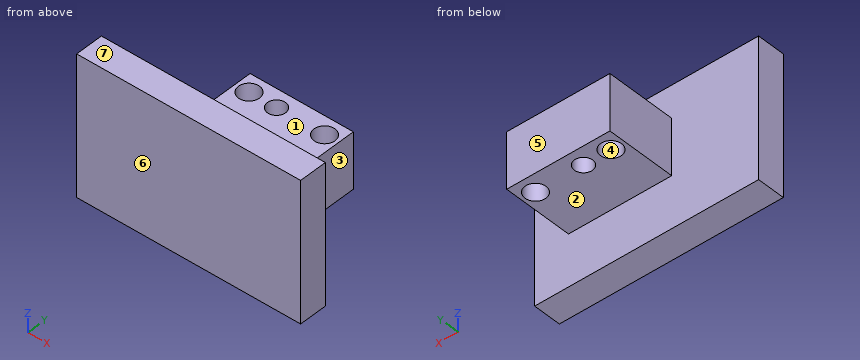
from build123d import *

# Parameters (mm, degrees)
SKETCH1_W           = 80
SKETCH1_H           = 50
MAIN_PLATE_DEPTH    = 10
SKETCH1_3_W         = 36.871622478
SKETCH1_3_H         = 20
BOSS_EXTRUDE2_DEPTH = 25
SKETCH2_R           = 3.760980907
SKETCH2_R_2         = 3.25
CUT_EXTRUDE1_DEPTH  = 20


with BuildPart() as part:
    # Sketch1 → Main Plate (new body)
    with BuildSketch(Plane(origin=(0, 0, 0), x_dir=(1, 0, 0), z_dir=(0, 1, 0))):
        Rectangle(SKETCH1_W, SKETCH1_H)
    extrude(amount=-MAIN_PLATE_DEPTH)

    # Sketch1<3> → Boss-Extrude2 (add)
    with BuildSketch(Plane(origin=(0, 0, 0), x_dir=(1, 0, 0), z_dir=(0, 1, 0))):
        with Locations((9.470325945, -3.44765343)):
            Rectangle(SKETCH1_3_W, SKETCH1_3_H)
    extrude(amount=BOSS_EXTRUDE2_DEPTH)

    # Sketch2 → Cut-Extrude1 (cut)
    with BuildSketch(Plane.XY.offset(13.44765343)):
        with Locations((-4.018286342, 18.961248544)):
            Circle(SKETCH2_R)
        with Locations(Location((22.958938232, 18.961248544, 0), (0, 0, 180))):
            Circle(SKETCH2_R)
        with Locations((5.79860133, 18.961248544)):
            Circle(SKETCH2_R_2)
    extrude(amount=-CUT_EXTRUDE1_DEPTH, mode=Mode.SUBTRACT)


solid = part.part
The listing builds one solid part. Answer for the finished solid, in the listing's coordinates (mm). Face numbers are marked on the shaded views. A direction names the side the tool comes from. Give positions to 0.01 mm unless a question says otherwise; leave off trailing zeros. Order: outer loops, then holes, each group sorted by start corner. A loop starts at its lowest first (then second) coordinate and runs counter-clockwise, first axis right, second up. Notation, with made-up numbers: (85.25, 60) -> (137.25, 60) arc R22 ccw to (137.25, 92) -> close; hole circle Ø11 at (-5.75, 28). An arc over 180 degrees is marked (long way). Put each result on its own line as item: value.
Item 1: For a pull along Y with two mould halves and no side action, classify the marked faces 4, 5, 6 and 7 as released by +Y, released by -Y, zero draft, split by the parting line, or undercut.
Established:
face 4: undercut
face 5: released by +Y
face 6: released by -Y
face 7: zero draft
Item 2: A cutting plane is placed at D-D on x = 14.5. Give the vertices of the cut face in (y, z).
Established:
outline: (-10, -25) -> (0, -25) -> (0, -6.55) -> (25, -6.55) -> (25, 13.45) -> (0, 13.45) -> (0, 25) -> (-10, 25) -> close
Item 3: A cutting plane is placed at A-A on x = -4. Give the vertices of the cut face in (y, z), plus the area to 3 significant figures.
Established:
outline: (-10, -25) -> (0, -25) -> (0, -6.55) -> (15.2, -6.55) -> (15.2, 13.45) -> (0, 13.45) -> (0, 25) -> (-10, 25) -> close; (22.72, -6.55) -> (25, -6.55) -> (25, 13.45) -> (22.72, 13.45) -> close
area: 850 mm^2
Item 4: Straight lines are drawn through the part: line 1 (X direction, y = 7.5, z = 9); line 2 (Z direction, x = -4, y = 7); line 3 (Y direction, x = 34, z = 8.5). For each, find the intervals that lie inside material, in ascending order.
Established:
line 1: x = -8.97 to 27.91
line 2: z = -6.55 to 13.45
line 3: y = -10 to 0
Item 5: For the marked faces 1, 2 and 3, determine the directions among +Z, -Z, +X, -X, +Y, -Y from which every point of the face is accessible in a straight line to the end or side of a thin tool.
Established:
face 1: +Z, +X, -X, +Y
face 2: -Z, +X, -X, +Y
face 3: +Z, -Z, +X, +Y
Item 6: Given P1, Ø12, axis at x = -4.02, y = 18.96, coming from the -Z side; P2, Ø2, axis at x = 15, z = -8, coming from the +Y side; P3, Ø10, axis at y = 10.5, z = 8, coming from the +X side, each flat-ended and moving along its own axis, determine where each tip first touches the part or whether it passes through.
Established:
P1: stops at z = -6.55
P2: stops at y = 0
P3: stops at x = 27.91
Item 7: A cutting plane is placed at B-B on y = 20. Give the vertices of the cut face in (x, z).
Established:
outline: (-8.97, -6.55) -> (-7.63, -6.55) -> (-7.63, 13.45) -> (-8.97, 13.45) -> close; (-0.4, -6.55) -> (2.72, -6.55) -> (2.72, 13.45) -> (-0.4, 13.45) -> close; (8.88, -6.55) -> (19.34, -6.55) -> (19.34, 13.45) -> (8.88, 13.45) -> close; (26.57, -6.55) -> (27.91, -6.55) -> (27.91, 13.45) -> (26.57, 13.45) -> close
Item 8: A cutting plane is placed at C-C on z = -1.5. Give the vertices of the cut face in (x, y).
Established:
outline: (-40, -10) -> (40, -10) -> (40, 0) -> (27.91, 0) -> (27.91, 25) -> (-8.97, 25) -> (-8.97, 0) -> (-40, 0) -> close; hole circle Ø7.52 at (-4.02, 18.96); hole circle Ø6.5 at (5.8, 18.96); hole circle Ø7.52 at (22.96, 18.96)
